from build123d import *

# Parameters (mm, degrees)
SKETCH_1_R      = 2.5
EXTRUDE_1_DEPTH = 10
EXTRUDE_2_DEPTH = 1


with BuildPart() as part:
    # 스케치1 → 보스-돌출1 (new body)
    with BuildSketch(Plane.XY):
        Circle(SKETCH_1_R)
    extrude(amount=EXTRUDE_1_DEPTH)

    # 스케치2 → 보스-돌출2 (add)
    with BuildSketch(Plane.XY.offset(10)):
        with BuildLine():
            ThreePointArc((-2.425994905, 0.603778702), (-2.165063509, 1.25), (-1.735885147, 1.799083866))
            Line((-1.735885147, 1.799083866), (-3.116104663, 1.799083866))
            Line((-3.116104663, 1.799083866), (-2.425994905, 0.603778702))
        make_face()
        with BuildLine():
            Line((-2.077403109, 0), (-1.038701554, 1.799083866))
            Line((-1.038701554, 1.799083866), (-1.735885147, 1.799083866))
            ThreePointArc((-1.735885147, 1.799083866), (-2.165063509, 1.25), (-2.425994905, 0.603778702))
            Line((-2.425994905, 0.603778702), (-2.077403109, 0))
        make_face()
        with BuildLine():
            Line((-1.038701554, 1.799083866), (1.038701554, 1.799083866))
            Line((1.038701554, 1.799083866), (0.690109758, 2.402862568))
            ThreePointArc((0.690109758, 2.402862568), (0, 2.5), (-0.690109758, 2.402862568))
            Line((-0.690109758, 2.402862568), (-1.038701554, 1.799083866))
        make_face()
        with BuildLine():
            Line((2.425994905, 0.603778702), (3.116104663, 1.799083866))
            Line((3.116104663, 1.799083866), (1.735885147, 1.799083866))
            ThreePointArc((1.735885147, 1.799083866), (2.165063509, 1.25), (2.425994905, 0.603778702))
        make_face()
        with BuildLine():
            ThreePointArc((2.425994905, 0.603778702), (2.165063509, 1.25), (1.735885147, 1.799083866))
            Line((1.735885147, 1.799083866), (1.038701554, 1.799083866))
            Line((1.038701554, 1.799083866), (2.077403109, 0))
            Line((2.077403109, 0), (2.425994905, 0.603778702))
        make_face()
        with BuildLine():
            Line((3.116104663, -1.799083866), (2.425994905, -0.603778702))
            ThreePointArc((2.425994905, -0.603778702), (2.165063509, -1.25), (1.735885147, -1.799083866))
            Line((1.735885147, -1.799083866), (3.116104663, -1.799083866))
        make_face()
        with BuildLine():
            Line((2.425994905, -0.603778702), (2.077403109, 0))
            Line((2.077403109, 0), (1.038701554, -1.799083866))
            Line((1.038701554, -1.799083866), (1.735885147, -1.799083866))
            ThreePointArc((1.735885147, -1.799083866), (2.165063509, -1.25), (2.425994905, -0.603778702))
        make_face()
        with BuildLine():
            Line((0, -3.598167732), (0.690109758, -2.402862568))
            ThreePointArc((0.690109758, -2.402862568), (0, -2.5), (-0.690109758, -2.402862568))
            Line((-0.690109758, -2.402862568), (0, -3.598167732))
        make_face()
        with BuildLine():
            Line((0.690109758, -2.402862568), (1.038701554, -1.799083866))
            Line((1.038701554, -1.799083866), (-1.038701554, -1.799083866))
            Line((-1.038701554, -1.799083866), (-0.690109758, -2.402862568))
            ThreePointArc((-0.690109758, -2.402862568), (0, -2.5), (0.690109758, -2.402862568))
        make_face()
        with BuildLine():
            Line((-1.038701554, -1.799083866), (-2.077403109, 0))
            Line((-2.077403109, 0), (-2.425994905, -0.603778702))
            ThreePointArc((-2.425994905, -0.603778702), (-2.165063509, -1.25), (-1.735885147, -1.799083866))
            Line((-1.735885147, -1.799083866), (-1.038701554, -1.799083866))
        make_face()
        with BuildLine():
            ThreePointArc((-1.735885147, -1.799083866), (-2.165063509, -1.25), (-2.425994905, -0.603778702))
            Line((-2.425994905, -0.603778702), (-3.116104663, -1.799083866))
            Line((-3.116104663, -1.799083866), (-1.735885147, -1.799083866))
        make_face()
        Polygon((0, -3.598167732), (3.116104663, 1.799083866), (-3.116104663, 1.799083866), align=None)
        Polygon((3.116104663, -1.799083866), (0, 3.598167732), (-3.116104663, -1.799083866), align=None)
        with BuildLine():
            ThreePointArc((-0.690109758, 2.402862568), (0, 2.5), (0.690109758, 2.402862568))
            Line((0.690109758, 2.402862568), (0, 3.598167732))
            Line((0, 3.598167732), (-0.690109758, 2.402862568))
        make_face()
    extrude(amount=EXTRUDE_2_DEPTH)


solid = part.part
For this review, take the finished solid that the model builds, in its own axes (mm). A direction names the side the tool comes from. Round coordinates to 2 decimals unless told otherwise and drop trailing zeros. Loops run counter-clockwise (first coordinate to the right, second up) from the corner with the lowest first, then second, coordinate; pieces in that order, holes last. Notation, with made-up numbers: (48, 6.25) - (106, 6.25) arc R28 ccw to (106, 39.25) - close; hole circle Ø7 at (56.5, 23). An arc over 180 degrees is marked (long way). Use one line per item in the form item = value.
Item 1: Consider section A-A on x = -0.25. Write out the cut boundary in (y, z).
Answers:
outline = (-3.17, 10) - (-2.49, 10) - (-2.49, 0) - (2.49, 0) - (2.49, 10) - (3.17, 10) - (3.17, 11) - (-3.17, 11) - close
Item 2: Consider section D-D on x = -2.25. Write out the cut boundary in (y, z), then the cut area to 3 significant figures.
Answers:
outline = (-1.8, 10) - (-1.09, 10) - (-1.09, 0) - (1.09, 0) - (1.09, 10) - (1.8, 10) - (1.8, 11) - (0.3, 11) - (0.3, 10) - (-0.3, 10) - (-0.3, 11) - (-1.8, 11) - close
area = 24.8 mm^2
Item 3: Clearance check with flat-ended pins moving along their axes: P1, Ø1, axis at x = 2, y = 1, coming from the -Z side; P2, Ø0.5, axis at x = 2, z = 10.5, coming from the +Y side; P3, Ø0.6, axis at x = -2.5, y = -1.5, coming from the -Z side; P4, Ø2, axis at x = 0, z = 1, coming from the -Y side. State where each tip first meets the part, or that it passes through.
Answers:
P1 = 0
P2 = 1.8
P3 = 10
P4 = -2.5
Item 4: Consider section C-C on z = 1. Write out the cut boundary in (x, y).
Answers:
outline = circle Ø5 at (0, 0)
Item 5: For line 1 (Y direction, x = 0, z = 6.25); line 2 (Z direction, x = 0, y = -3); line 3 (X direction, y = -1.25, z = 6.25), list the stretches that pass through material, from the lowest coordinate up.
Answers:
line_1 = -2.5 to 2.5
line_2 = 10 to 11
line_3 = -2.17 to 2.17
Item 6: Tool access review of faces 1 (the flat face through (2.1, 1.799, 10.5)), 2 (the flat face through (-2.1, 1.799, 10.5)), 3 (the flat face through (2.4, 1.5, 10)): name each direction out of +Z, -Z, +X, -X, +Y, -Y from which nothing blocks a thin tool from reaching the whole face with its end or side.
Answers:
face_1 = +Z, +X, +Y
face_2 = +Z, -X, +Y
face_3 = -Z, +X, +Y
Item 7: Consider section B-B on y = 2. Write out the cut boundary in (x, z).
Answers:
outline = (-1.5, 0) - (1.5, 0) - (1.5, 10) - (0.92, 10) - (0.92, 11) - (-0.92, 11) - (-0.92, 10) - (-1.5, 10) - close
